Build history of the part. All positions in model axes, mm. Face numbers are marked on the shaded views. A direction names the side the tool comes from. Round coordinates to 2 decimals unless told otherwise and drop trailing zeros. Write each loop counter-clockwise with the first axis right and the second up, starting at its lowest first coordinate (ties: lowest second). Pieces come first, ordered by that corner, then holes.
1) Flat gauge pins, fed straight in: pin 1 (3 mm diameter, centred on y = -66, z = 0.5, fed in from +X); pin 2 (3 mm diameter, centred on x = 0, z = 8.5, fed in from -Y); pin 3 (2.5 mm diameter, centred on y = -75, z = 4.5, fed in from -X); pin 4 (6 mm diameter, centred on y = -84, z = -8, fed in from +X). Where does each tip first touch, or does it go through?
2) Which spindle directions (+Z, -Z, +X, -X, +Y, -Y) get a long thin tool onto all of the face, cutting with end or side? Do the marked faces 1, 2 and 3. Say none if no direction does.
3) Pull direction Z, two halves, no side cores. Call the marked faces 4, 5 and 6: +Z half, -Z half, draft (parallel to the pull), parting line (faces both ways), or undercut.
4) Saw through at D-D (x = 20.5). Write the cut outline in (y, z).
5) Wall check: probe 1 along Y at (x, z) = (20.5, 12.95); probe 2 along X at (y, z) = (-83, 13.95); probe 3 along Y at (x, z) = (-20, 13). Give the ranges that are in metal, low to high.
6) Saw through at C-C (z = -3). Write the cut outline in (x, y).
7) Saw through at A-A (y = -74.5). Write the cut outline in (x, z).
8) Saw through at B-B (x = 0). Write the cut outline in (y, z), plus the area to 3 significant figures.
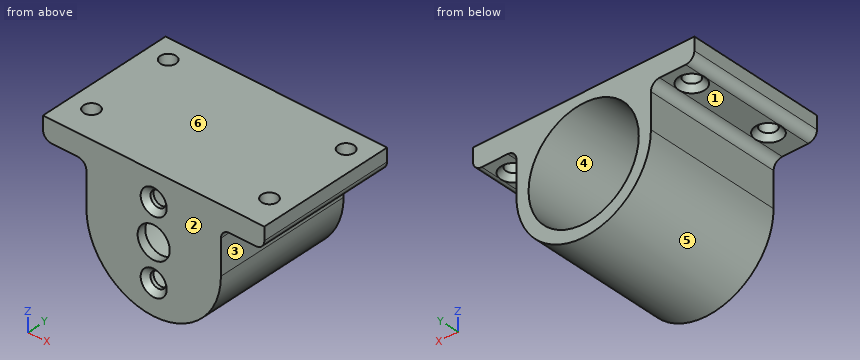
from build123d import *

# Parameters (mm, degrees)
PAD001_START    = 60
PAD001_DEPTH    = 32
SKETCH002_R     = 12.7
POCKET_DEPTH    = 30
SKETCH003_R     = 1.8
SKETCH003_R_2   = 3.7
POCKET001_DEPTH = 2
SKETCH004_R     = 1.8
POCKET002_DEPTH = 5.001
SKETCH010_R     = 3
POCKET006_DEPTH = 1.2
POCKET006_TAPER = 45
SKETCH033_R     = 3
POCKET020_DEPTH = 2
POCKET020_TAPER = 45


with BuildPart() as part:
    # Sketch001 → Pad001 (new body)
    with BuildSketch(Plane.XZ.offset(PAD001_START)):
        with BuildLine():
            ThreePointArc((-15.5, 0), (0, -15.5), (15.5, 0))
            Line((15.5, 8), (15.5, 0))
            ThreePointArc((17.5, 10), (16.085786, 9.414214), (15.5, 8))
            Line((23.5, 10), (17.5, 10))
            ThreePointArc((23.5, 10), (24.914214, 10.585786), (25.5, 12))
            Line((25.5, 15), (25.5, 12))
            Line((-25.5, 15), (25.5, 15))
            Line((-25.5, 12), (-25.5, 15))
            ThreePointArc((-25.5, 12), (-24.914214, 10.585786), (-23.5, 10))
            Line((-17.5, 10), (-23.5, 10))
            ThreePointArc((-15.5, 8), (-16.085786, 9.414214), (-17.5, 10))
            Line((-15.5, 0), (-15.5, 8))
        make_face()
    extrude(amount=PAD001_DEPTH)

    # Sketch002 (on Face13 of Pad001) → Pocket (cut)
    with BuildSketch(Plane(origin=(0, -60, 0), x_dir=(1, 0, 0), z_dir=(0, 1, 0))):
        Circle(SKETCH002_R)
    extrude(amount=-POCKET_DEPTH, mode=Mode.SUBTRACT)

    # Sketch003 (on Face5 of Pocket) → Pocket001 (cut)
    with BuildSketch(Plane.XZ.offset(92)):
        with Locations((0, 8.5)):
            Circle(SKETCH003_R)
        with Locations((0, -8.5)):
            Circle(SKETCH003_R)
        Circle(SKETCH003_R_2)
    extrude(amount=-POCKET001_DEPTH, mode=Mode.SUBTRACT)

    # Sketch004 (on Face3 of Pocket001) → Pocket002 (cut, through all)
    with BuildSketch(Plane(origin=(0, 0, 10), x_dir=(1, 0, 0), z_dir=(0, 0, -1))):
        with Locations((-20.5, 85)):
            Circle(SKETCH004_R)
        with Locations((-20.5, 65)):
            Circle(SKETCH004_R)
        with Locations((20.5, 65)):
            Circle(SKETCH004_R)
        with Locations((20.5, 85)):
            Circle(SKETCH004_R)
    extrude(amount=-POCKET002_DEPTH, mode=Mode.SUBTRACT)

    # Sketch010 (on Face3 of Pocket002) → Pocket006 (cut)
    with BuildSketch(Plane(origin=(0, 0, 10), x_dir=(1, 0, 0), z_dir=(0, 0, -1))):
        with Locations((-20.5, 85)):
            Circle(SKETCH010_R)
        with Locations((20.5, 85)):
            Circle(SKETCH010_R)
        with Locations((20.5, 65)):
            Circle(SKETCH010_R)
        with Locations((-20.5, 65)):
            Circle(SKETCH010_R)
    extrude(amount=-POCKET006_DEPTH, taper=POCKET006_TAPER, mode=Mode.SUBTRACT)

    # Sketch033 (on Face7 of Pocket006) → Pocket020 (cut)
    with BuildSketch(Plane.XZ.offset(92)):
        with Locations((0, 8.5)):
            Circle(SKETCH033_R)
        with Locations((0, -8.5)):
            Circle(SKETCH033_R)
    extrude(amount=-POCKET020_DEPTH, taper=POCKET020_TAPER, mode=Mode.SUBTRACT)


with BuildPart() as part_1:
    # Body001 placement: moved
    add(part.part.moved(Location((0, 2, 0))))


solid = part_1.part
Evaluation:
1. pin 1: stops at x = 15.5
1. pin 2: passes through
1. pin 3: stops at x = -15.5
1. pin 4: stops at x = 14.67
2. face 1: -Z, -X, +Y, -Y
2. face 2: +Z, -Z, +X, -X, -Y
2. face 3: -Z, +X, +Y, -Y
3. face 4: undercut
3. face 5: -Z half
3. face 6: +Z half
4. outline: (-90, 10) - (-86, 10) - (-84.8, 11.2) - (-84.8, 15) - (-90, 15) - close; (-81.2, 11.2) - (-80, 10) - (-66, 10) - (-64.8, 11.2) - (-64.8, 15) - (-81.2, 15) - close; (-61.2, 11.2) - (-60, 10) - (-58, 10) - (-58, 15) - (-61.2, 15) - close
5. probe 1: y = -90 to -84.8, -81.2 to -64.8, -61.2 to -58
5. probe 2: x = -25.5 to -22.3, -18.7 to 18.7, 22.3 to 25.5
5. probe 3: y = -90 to -84.73, -81.27 to -64.73, -61.27 to -58
6. outline: (-15.21, -90) - (-2.17, -90) - (-2.17, -88) - (-12.34, -88) - (-12.34, -58) - (-15.21, -58) - close; (2.17, -90) - (15.21, -90) - (15.21, -58) - (12.34, -58) - (12.34, -88) - (2.17, -88) - close
7. outline: (-25.5, 12) arc R2 ccw to (-23.5, 10) - (-17.5, 10) arc R2 cw to (-15.5, 8) - (-15.5, 0) arc R15.5 ccw to (15.5, 0) - (15.5, 8) arc R2 cw to (17.5, 10) - (23.5, 10) arc R2 ccw to (25.5, 12) - (25.5, 15) - (-25.5, 15) - close; hole circle Ø25.4 at (0, 0)
8. outline: (-90, -15.5) - (-58, -15.5) - (-58, -12.7) - (-88, -12.7) - (-88, -10.3) - (-88.8, -10.3) - (-90, -11.5) - close; (-90, -5.5) - (-88.8, -6.7) - (-88, -6.7) - (-88, -3.7) - (-90, -3.7) - close; (-90, 3.7) - (-88, 3.7) - (-88, 6.7) - (-88.8, 6.7) - (-90, 5.5) - close; (-90, 11.5) - (-88.8, 10.3) - (-88, 10.3) - (-88, 12.7) - (-58, 12.7) - (-58, 15) - (-90, 15) - close
8. area: 182 mm2
